Input: part model. Units: mm. Frame: model coordinates. Face numbers are marked on the shaded views. A direction names the side the tool comes from. Round coordinates to 2 decimals unless told otherwise and drop trailing zeros. Write each loop counter-clockwise with the first axis right and the second up, starting at its lowest first coordinate (ties: lowest second). Pieces come first, ordered by that corner, then holes. Notation, with made-up numbers: (75, 63) -> (97, 63) arc R16 ccw to (97, 75) -> close; hole circle Ø4 at (57, -17). An arc over 180 degrees is marked (long way). Write item = value, one per line.
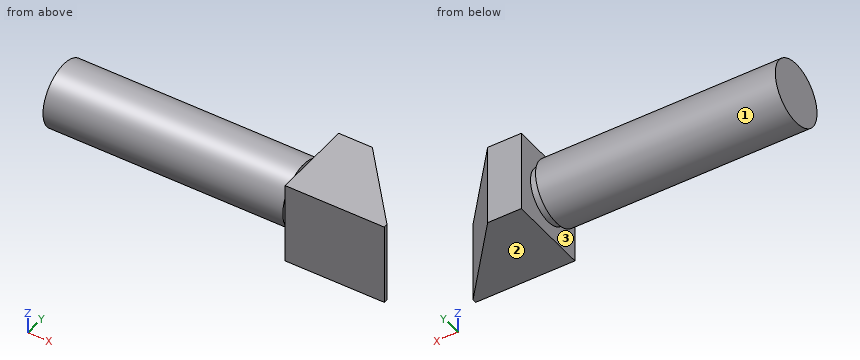
```python
from build123d import *

# Parameters (mm, degrees)
SKETCH1_R           = 3.85
BOSS_EXTRUDE1_DEPTH = 30
SKETCH2_R           = 3.85
SKETCH2_R_2         = 3.25
CUT_EXTRUDE1_DEPTH  = 1
SKETCH3_W           = 9.9
SKETCH3_H           = 9.9
BOSS_EXTRUDE2_DEPTH = 12
CUT_EXTRUDE2_DEPTH  = 12


with BuildPart() as part:
    # Sketch1 → Boss-Extrude1 (new body)
    with BuildSketch(Plane(origin=(0, 0, 0), x_dir=(0, 0, -1), z_dir=(1, 0, 0))):
        Circle(SKETCH1_R)
    extrude(amount=BOSS_EXTRUDE1_DEPTH)

    # Sketch2 → Cut-Extrude1 (cut)
    with BuildSketch(Plane(origin=(30, 0, 0), x_dir=(0, 0, -1), z_dir=(1, 0, 0))):
        Circle(SKETCH2_R)
        Circle(SKETCH2_R_2, mode=Mode.SUBTRACT)
    extrude(amount=-CUT_EXTRUDE1_DEPTH, mode=Mode.SUBTRACT)

    # Sketch3 → Boss-Extrude2 (add)
    with BuildSketch(Plane(origin=(30, 0, 0), x_dir=(0, 0, -1), z_dir=(1, 0, 0))):
        Rectangle(SKETCH3_W, SKETCH3_H)
    extrude(amount=BOSS_EXTRUDE2_DEPTH)

    # Sketch4 → Cut-Extrude2 (cut)
    with BuildSketch(Plane.XY.offset(4.95)):
        Polygon((34.067156878, 4.95), (42, -4.45), (42, 4.95), align=None)
    extrude(amount=-CUT_EXTRUDE2_DEPTH, mode=Mode.SUBTRACT)


solid = part.part
```
1) Cut plane C-C (x = 18). Return the cut outline in (y, z), and give its area (3 significant figures).
Solutions:
outline = circle Ø7.7 at (0, 0)
area = 46.6 mm^2
2) Cut plane B-B (y = 2.75). Return the cut outline in (x, z).
Solutions:
outline = (0, -2.69) -> (29, -2.69) -> (29, -1.73) -> (30, -1.73) -> (30, -4.95) -> (35.92, -4.95) -> (35.92, 4.95) -> (30, 4.95) -> (30, 1.73) -> (29, 1.73) -> (29, 2.69) -> (0, 2.69) -> close
3) Cut plane A-A (z = 0). Return the cut outline in (x, y), and give its area (3 significant figures).
Solutions:
outline = (0, -3.85) -> (29, -3.85) -> (29, -3.25) -> (30, -3.25) -> (30, -4.95) -> (42, -4.95) -> (42, -4.45) -> (34.07, 4.95) -> (30, 4.95) -> (30, 3.25) -> (29, 3.25) -> (29, 3.85) -> (0, 3.85) -> close
area = 311 mm^2
4) First-contact query: P1, Ø1.5, axis at x = 25.5, y = 2, coming from the -Z side; P2, Ø1, axis at y = -0.5, z = -3, coming from the -X side; P3, Ø4, axis at x = 5, y = -1.5, coming from the -Z side; P4, Ø3, axis at y = -1, z = -3, coming from the +X side. Flat tips, straight axial feed; report the tip coordinate or a pass-through.
Solutions:
P1 = -3.64
P2 = 0
P3 = -3.85
P4 = 40.35
5) Line query: L1, parallel to X at y = -3.75, z = 0.5; L2, parallel to X at y = -2, z = 2.75; L3, parallel to Z at x = 13, y = 0.25. Output: solid intervals per line, ascending. Write a range as from..to.
Solutions:
L1 = 0..29, 30..41.41
L2 = 0..29, 30..39.93
L3 = -3.84..3.84
6) Cut plane D-D (z = 2.5). Return the cut outline in (x, y).
Solutions:
outline = (0, -2.93) -> (29, -2.93) -> (29, -2.08) -> (30, -2.08) -> (30, -4.95) -> (42, -4.95) -> (42, -4.45) -> (34.07, 4.95) -> (30, 4.95) -> (30, 2.08) -> (29, 2.08) -> (29, 2.93) -> (0, 2.93) -> close
7) Access query for the marked faces 1, 2 and 3. Directions: +Z, -Z, +X, -X, +Y, -Y. A direction counts if a zero-diameter tool reaches every point of the face in a straight line with its end or side. Return the directions, or none.
Solutions:
face_1 = -X
face_2 = -Z, +X, -X, +Y, -Y
face_3 = none
